Source: CAD feature listing. Evaluate the final solid. Frame: model axes, mm. A direction names the side the tool comes from. Coordinates: 2 decimals unless noted, no trailing zeros. Order: outer loops, then holes, each group sorted by start corner. A loop starts at its lowest first (then second) coordinate and runs counter-clockwise, first axis right, second up.
Item 1: Section A-A on z = 18.75. Return the cut outline in (x, y), then the cut area to 3 significant figures.
Item 2: Reachability of faces 4 (the flat face through (-10.874, 39.158, 13.339)), 5 (the cylindrical face through (-1, 15, 2)) from +Z, -Z, +X, -X, +Y, -Y: full face, straight path, thin tool, end or side. Return the list, or none.
Item 3: Contact query for flat-ended pins moving along their axis: P1, Ø2, axis at x = -16, y = 1, coming from the +Z side; P2, Ø5, axis at x = -32, z = 14.5, coming from the +Y side; P3, Ø6, axis at x = -5, z = 16, coming from the -Y side. Output: stop coordinate, or through.
Item 4: Section B-B on y = 16. Return the cut outline in (x, z), then the cut area to 3 significant figures.
Item 5: Ray query, line 1 (X direction, y = 26, z = 12); line 2 (Z direction, x = -19.5, y = 9.5); line 3 (X direction, y = 43, z = 8.5). Return the intervals inside material, ascending.
Item 6: Mould query, pull axis Y, two halves, no side actions, for faces 1 (the cylindrical face through (-31.452, -5.638, 1.504)), 2 (the flat face through (-20, 19, 0)), 3 (the flat face through (-8.974, -5.248, 13.339)). Classes: released by +Y, released by -Y, zero draft, split by the parting line, or undercut.
from build123d import *

# Parameters (mm, degrees)
F0_W     = 40
F0_H     = 30
F1_DEPTH = 25
F2_T     = -2
F3_R     = 5


with BuildPart() as f1:
    # F0 (on Top) → F1 (new body)
    with BuildSketch(Plane.XY):
        Polygon((0, 30), (-20, 52.36068), (-40, 30), align=None)
        with Locations((-20, 15)):
            Rectangle(F0_W, F0_H)
        Polygon((0, 0), (-40, 0), (-25, -13.228757), (-15, -13.228757), align=None)
    extrude(amount=F1_DEPTH)

    # F2
    f2_openings = [f1.faces().sort_by_distance(p)[0] for p in [
        (-20, 16.683957, 25),
    ]]
    offset(amount=F2_T, openings=f2_openings)

    # F3
    f3_edges = [f1.edges().sort_by_distance(p)[0] for p in [
        (-40, 15, 0),
        (-30, 41.18034, 0),
        (-10, 41.18034, 0),
        (0, 15, 0),
        (-32.5, -6.614378, 0),
        (-7.5, -6.614378, 0),
        (-20, -13.228757, 0),
    ]]
    fillet(f3_edges, radius=F3_R)


solid = f1.part
Answer list:
1. outline: (-40, 0) - (-25, -13.23) - (-15, -13.23) - (0, 0) - (0, 30) - (-20, 52.36) - (-40, 30) - close; hole (-38, 0.9) - (-24.24, -11.23) - (-15.76, -11.23) - (-2, 0.9) - (-2, 29.24) - (-20, 49.36) - (-38, 29.24) - close
1. area: 326 mm2
2. face 4: +Z
2. face 5: -Z, +X, +Y, -Y
3. P1: stops at z = 2
3. P2: stops at y = 41.74
3. P3: stops at y = -7.06
4. outline: (-40, 5) arc R5 ccw to (-35, 0) - (-5, 0) arc R5 ccw to (0, 5) - (0, 25) - (-2, 25) - (-2, 2) - (-38, 2) - (-38, 25) - (-40, 25) - close
4. area: 161 mm2
5. line 1: x = -40 to -38, -2 to 0
5. line 2: z = 0 to 2
5. line 3: x = -28.37 to -25.69, -14.31 to -11.63
6. face 1: released by -Y
6. face 2: zero draft
6. face 3: undercut
